Can you work these out from the model? Positions are in its coordinate system, mm. A direction names the side the tool comes from. Coordinates: 2 decimals unless noted, no trailing zeros. Order: outer loops, then holes, each group sorted by start corner. A loop starts at its lowest first (then second) coordinate and runs counter-clockwise, first axis right, second up. Notation, with made-up numbers: (17, 22.5) -> (52, 22.5) arc R10 cw to (52, 26.5) -> close; hole circle Ø11 at (-39, 39). An arc over 180 degrees is marked (long way). Answer in a Markdown table with one row per item. Add a question column.
1. We'd pull the mould along Y, two halves only. Please class faces 4 (the face through (-18.175, 38, 2)), 5 (the face through (0.035, -39.413, 1.61)): pulls with the +Y half, pulls with the -Y half, needs draft (parallel to the pull), parting line crosses it, or undercut.
2. Imagine slicing it at A-A on y = -75.5. Write out the boundary of the cut face in (x, z) (1 decimal), plus the area to 3 significant figures.
3. Imagine slicing it at C-C on y = -59. Write out the boundary of the cut face in (x, z) (3 decimals), plus the area to 4 significant figures.
4. Will this pin go through, and if not, where does the flat tip stop? pin 1 (1 mm diameter, centred on y = -67, z = 2, fed in from +X).
5. On a 3-axis mill with a long thin cutter (end or side, diameter ignored), from which of +Z, -Z, +X, -X, +Y, -Y can I reach the whole of each face in a straight line? I mean faces 1 (the face through (1.588, -72, 2)), 2 (the face through (-15, -33, 2)), 3 (the face through (17, -71, 2)). Say none if no direction works.
6. If I drill on line 1 along Y through (x, z) = (0, 2.3); line 2 along Y through (x, z) = (16, 2.3); line 3 along X through (y, z) = (-42, 1) (1 decimal), over which ranges is the centre line in solid material (lowest first)? Write a range as [from, to].
7. Imagine slicing it at B-B on x = 0. Write out the boundary of the cut face in (y, z) (1 decimal), plus the area to 3 significant figures.
8. Imagine slicing it at D-D on z = 2. State how many separate pieces and enclosed holes the cut face has, plus the area to 3 significant figures.
from build123d import *

# Parameters (mm, degrees)
F1_DEPTH  = 3.175
F1_FACE_W = 30
F1_FACE_H = 3.175
F2_DEPTH  = 45
F3_R      = 4
F3_W      = 3.175
F3_H      = 10
F4_DEPTH  = 25
F5_W      = 15
F5_H      = 3.175
F6_DEPTH  = 3.175
F7_W      = 15
F7_H      = 3.175
F8_DEPTH  = 3.175


with BuildPart() as f1:
    # F0 (on Top) → F1 (new body)
    with BuildSketch(Plane.XY):
        Polygon((-15, -41), (15, -41), (15, -26), (18.175, -26), (18.175, -11), (15, -11), (15, 4), (18.175, 4), (18.175, 19), (15, 19), (15, 34), (18.175, 34), (18.175, 41), (-18.175, 41), (-18.175, 34), (-15, 34), (-15, 19), (-18.175, 19), (-18.175, 4), (-15, 4), (-15, -11), (-18.175, -11), (-18.175, -26), (-15, -26), align=None)
    extrude(amount=F1_DEPTH)

    # F1_face (on face) → F2 (join)
    with BuildSketch(Plane(origin=(0, -41, 1.5875), x_dir=(1, 0, 0), z_dir=(0, -1, 0))):
        Rectangle(F1_FACE_W, F1_FACE_H)
    extrude(amount=F2_DEPTH)

    # F3 (on face) → F4 (cut)
    with BuildSketch(Plane.XY.offset(3.175)):
        with Locations((0, -59)):
            Circle(F3_R)
        with BuildLine():
            ThreePointArc((-1.5875, -51), (0, -52.5875), (1.5875, -51))
            Line((1.5875, -51), (-1.5875, -51))
        make_face()
        with Locations((0, -46)):
            Rectangle(F3_W, F3_H)
        with BuildLine():
            Line((-1.5875, -41), (1.5875, -41))
            ThreePointArc((1.5875, -41), (0, -39.4125), (-1.5875, -41))
        make_face()
        with BuildLine():
            ThreePointArc((-1.5875, -77), (0, -78.5875), (1.5875, -77))
            Line((1.5875, -77), (-1.5875, -77))
        make_face()
        with Locations((0, -72)):
            Rectangle(F3_W, F3_H)
        with BuildLine():
            Line((-1.5875, -67), (1.5875, -67))
            ThreePointArc((1.5875, -67), (0, -65.4125), (-1.5875, -67))
        make_face()
    extrude(amount=-F4_DEPTH, mode=Mode.SUBTRACT)

    # F5 (on face) → F6 (join)
    with BuildSketch(Plane.YZ.offset(15)):
        with Locations((-78.5, 1.5875)):
            Rectangle(F5_W, F5_H)
        with Locations((-48.5, 1.5875)):
            Rectangle(F5_W, F5_H)
    extrude(amount=F6_DEPTH)

    # F7 (on face) → F8 (join)
    with BuildSketch(Plane(origin=(-15, 0, 0), x_dir=(0, -1, 0), z_dir=(-1, 0, 0))):
        with Locations((48.5, 1.5875)):
            Rectangle(F7_W, F7_H)
        with Locations((78.5, 1.5875)):
            Rectangle(F7_W, F7_H)
    extrude(amount=F8_DEPTH)


solid = f1.part
Answers follow:
| question | item | result |
|---|---|---|
| 1 | face 4 | needs draft |
| 1 | face 5 | undercut |
| 2 | outline | (-18.2, 0) -> (-1.6, 0) -> (-1.6, 3.2) -> (-18.2, 3.2) -> close; (1.6, 0) -> (18.2, 0) -> (18.2, 3.2) -> (1.6, 3.2) -> close |
| 2 | area | 105 mm² |
| 3 | outline | (-15, 0) -> (-4, 0) -> (-4, 3.175) -> (-15, 3.175) -> close; (4, 0) -> (15, 0) -> (15, 3.175) -> (4, 3.175) -> close |
| 3 | area | 69.85 mm² |
| 4 | pin 1 | stops at x = 15 |
| 5 | face 1 | +Z, -Z |
| 5 | face 2 | +Z, -Z, -X |
| 5 | face 3 | +Z, -Z, +X |
| 6 | line 1 | y = [-86, -78.59], [-65.41, -63], [-55, -52.59], [-39.41, 41] |
| 6 | line 2 | y = [-86, -71], [-56, -41], [-26, -11], [4, 19], [34, 41] |
| 6 | line 3 | x = [-18.2, -1.6], [1.6, 18.2] |
| 7 | outline | (-86, 0) -> (-78.6, 0) -> (-78.6, 3.2) -> (-86, 3.2) -> close; (-65.4, 0) -> (-63, 0) -> (-63, 3.2) -> (-65.4, 3.2) -> close; (-55, 0) -> (-52.6, 0) -> (-52.6, 3.2) -> (-55, 3.2) -> close; (-39.4, 0) -> (41, 0) -> (41, 3.2) -> (-39.4, 3.2) -> close |
| 7 | area | 294 mm² |
| 8 | separate pieces | 1 |
| 8 | enclosed holes | 3 |
| 8 | area | 4,110 mm² |
